Geometry: final body of the model. Coordinates: model frame, mm. Coordinates: 2 decimals unless noted, no trailing zeros. Loops run counter-clockwise (first coordinate to the right, second up) from the corner with the lowest first, then second, coordinate; pieces in that order, holes last. Notation, with made-up numbers: (-8.75, 84.25) - (12.25, 84.25) arc R8 cw to (12.25, 97.25) - close; hole circle Ø1 at (-4, 42.25). An arc over 180 degrees is marked (long way). Answer in a Markdown table with one row per item.
from build123d import *

# Parameters (mm, degrees)
F0_W     = 173.482
F0_H     = 106.426
F1_DEPTH = 14
F2_W     = 134.874
F2_H     = 81.295477
F3_DEPTH = 0.635
F4_R     = 5.715
F5_DEPTH = 25.4


with BuildPart() as f1:
    # F0 (on Front) → F1 (new body)
    with BuildSketch(Plane.XZ):
        with Locations((9.842499, 27.721002)):
            Rectangle(F0_W, F0_H)
    extrude(amount=F1_DEPTH)

    # F2 (on face) → F3 (cut)
    with BuildSketch(Plane.XZ.offset(14)):
        with Locations((9.842499, 27.71604)):
            Rectangle(F2_W, F2_H)
    extrude(amount=-F3_DEPTH, mode=Mode.SUBTRACT)

    # F4 (on face) → F5 (cut)
    with BuildSketch(Plane.XZ.offset(14)):
        with Locations((-76.898501, 80.934002)):
            Circle(F4_R)
        with Locations((-76.898501, -25.491998)):
            Circle(F4_R)
        with BuildLine():
            ThreePointArc((102.298499, -25.491998), (96.583499, -19.776998), (90.868499, -25.491998))
            ThreePointArc((90.868499, -25.491998), (96.583499, -31.206998), (102.298499, -25.491998))
        make_face()
        with BuildLine():
            ThreePointArc((102.298499, 80.934002), (96.583499, 86.649002), (90.868499, 80.934002))
            ThreePointArc((90.868499, 80.934002), (96.583499, 75.219002), (102.298499, 80.934002))
        make_face()
    extrude(amount=-F5_DEPTH, mode=Mode.SUBTRACT)


solid = f1.part
(1) Cut plane B-B on z = 11.5. Output: boundary loops of the cut face in (x, y) (1 decimal), then the cut area to 3 significant figures.
Verdict:
| item | result |
|---|---|
| outline | (-76.9, -14) - (-57.6, -14) - (-57.6, -13.4) - (77.3, -13.4) - (77.3, -14) - (96.6, -14) - (96.6, 0) - (-76.9, 0) - close |
| area | 2,340 mm² |
(2) First-contact query: pin 1 Ø10 at (x, z) = (28.5, 27) entering from -Y (3 decimals); pin 2 Ø4 at (x, z) = (76, 59.5) entering from -Y. Flat tips, straight axial feed; report the tip coordinate or a pass-through.
Verdict:
| item | result |
|---|---|
| pin 1 | stops at y = -13.365 |
| pin 2 | stops at y = -14 |
(3) Ray query, probe 1 along Y at (x, z) = (68, -9) (3 decimals). Return the intervals inside material, ascending.
Verdict:
| item | result |
|---|---|
| probe 1 | y = -13.365 to 0 |
(4) Pull-direction query (X, two-part tool) for faces 1 (the face through (92.587, -7.098, -21.407)), 2 (the face through (9, -13.365, 28)), 3 (the face through (9, -14, -19)), 4 (the face through (-76.899, -7, 27)); classes: pulls with the +X half, pulls with the -X half, needs draft (parallel to the pull), parting line crosses it, or undercut.
Verdict:
| item | result |
|---|---|
| face 1 | pulls with the +X half |
| face 2 | undercut |
| face 3 | needs draft |
| face 4 | pulls with the -X half |
(5) Cut plane A-A on x = -3.5. Output: boundary loops of the cut face in (y, z) (3 decimals), then the cut area to 3 significant figures.
Verdict:
| item | result |
|---|---|
| outline | (-14, -25.492) - (0, -25.492) - (0, 80.934) - (-14, 80.934) - (-14, 68.364) - (-13.365, 68.364) - (-13.365, -12.932) - (-14, -12.932) - close |
| area | 1,440 mm² |
